Autodesk Fusion 360 part; units mm, degrees
sketch "Skizze1" plane through (0, 0, 0) normal (0, 1, 0) x (1, 0, 0)
  line L0 (13.5, -1) -> (-13.5, -1)
  line L1 (-13.5, -1) -> (-13.5, 0)
  line L2 (-13.5, 0) -> (13.5, 0)
  line L3 (13.5, 0) -> (13.5, -1)
  line L4 (13.5, -1) -> (-13.5, 0) construction
  line L5 (-13.5, -1) -> (13.5, 0) construction
  line L6 (-13.5, 0) -> (-12.5, 0)
  line L7 (-12.5, 0) -> (-12.5, -7.5)
  line L8 (-12.5, -7.5) -> (-13.5, -7.5)
  line L9 (-13.5, -7.5) -> (-13.5, 0)
  line L10 (13.5, 0) -> (12.5, 0)
  line L11 (12.5, 0) -> (12.5, -7.5)
  line L12 (12.5, -7.5) -> (13.5, -7.5)
  line L13 (13.5, -7.5) -> (13.5, 0)
  line L14 (-12.5, -7.5) -> (-17.5, -7.5)
  line L15 (-17.5, -7.5) -> (-17.5, -6.5)
  line L16 (-17.5, -6.5) -> (-12.5, -6.5)
  line L17 (-12.5, -6.5) -> (-12.5, -7.5)
  line L18 (12.5, -7.5) -> (17.5, -7.5)
  line L19 (17.5, -7.5) -> (17.5, -6.5)
  line L20 (17.5, -6.5) -> (12.5, -6.5)
  line L21 (12.5, -6.5) -> (12.5, -7.5)
  point P0 (0, -0.5)
  dimension "d7" = 27
  dimension "d8" = 1
  dimension "d9" = 7.5
  dimension "d10" = 1
  dimension "d11" = 7.5
  dimension "d12" = 1
  dimension "d13" = 5
  dimension "d14" = 1
  dimension "d15" = 5
  dimension "d16" = 1
extrude "Extrusion1" add sketch "Skizze1" along normal blind 100
fillet "Abrundung1" radius 1.5 4 edges at (12.5, 50, 7.5) (-12.5, 50, 7.5) (13.5, 50, 0) (-13.5, 50, 0)
fillet "Abrundung2" radius 0.5 4 edges at (-13.5, 50, 6.5) (13.5, 50, 6.5) (12.5, 50, 1) (-12.5, 50, 1)
sketch "Skizze2" plane through (0, 0, 1) normal (0, 0, 1) x (-1, 0, 0)
  line L0 (12, -100) -> (12, 0)
  line L1 (12, 0) -> (-12, 0)
  line L2 (-12, 0) -> (-12, -100)
  line L3 (-12, -100) -> (12, -100)
  line L4 (0, 0) -> (0, -3.5) construction
  line L5 (-2.6, -6.1) -> (-2.6, -18.9)
  arc A0 (-2.6, -18.9) -> (2.6, -18.9) centre (0, -18.9) ccw
  line L6 (2.6, -18.9) -> (2.6, -6.1)
  arc A1 (2.6, -6.1) -> (-2.6, -6.1) centre (0, -6.1) ccw
  line L7 (0, -3.5) -> (0, -21.5) construction
  point P0 (0, -3.5)
  dimension "d26" = 3.5
  dimension "d34" = 18
  dimension "d35" = 5.2
extrude "Extrusion2" cut sketch "Skizze2" against normal blind 1 contours L5 A0 L6 A1
pattern_linear "R-Anordnung1" count 4 spacing 25 along (0, 1, 0) of "Extrusion2"
equation "InnerWidth = 27 mm"
equation "OuterWidth = 37 mm"
equation "Height = 7.5 mm"
equation "Thickness = 1 mm"
equation "Length = 100 mm"
equation "SlotDistance = 25 mm"
equation "d7 = InnerWidth"
equation "d8 = Thickness"
equation "d9 = Height"
equation "d10 = Thickness"
equation "d11 = Height"
equation "d12 = Thickness"
equation "d13 = ( OuterWidth - InnerWidth ) / 2"
equation "d14 = Thickness"
equation "d15 = ( OuterWidth - InnerWidth ) / 2"
equation "d16 = Thickness"
equation "d17 = Length"
equation "OuterFillet = 1.5 mm"
equation "d20 = OuterFillet"
equation "InnerFillet = OuterFillet - Thickness"
equation "d22 = InnerFillet"
equation "SlotWidth = 5.2 mm"
equation "SlotLength = 18 mm"
equation "SlotDistance2 = 25 mm"
equation "d26 = Linear Dimension-2"
equation "d30 = Length / SlotDistance2"
equation "d32 = SlotDistance2"
equation "d34 = SlotLength"
equation "d35 = SlotWidth"
Model file for the job. Use its own axes, mm. A direction names the side the tool comes from. Round coordinates to 2 decimals unless told otherwise and drop trailing zeros. Order: outer loops, then holes, each group sorted by start corner. A loop starts at its lowest first (then second) coordinate and runs counter-clockwise, first axis right, second up.
(1) Band-saw the part on B-B (y = 42). List the corners of the cut face in (x, z).
(2) 3-axis set-ups, long thin cutter, end or side, ignore diameter. For faces 1 (the face through (16, 49, 6.5)), 2 (the face through (-13.5, 49, 4)), 3 (the face through (-0.1, 28.5, 0.5)): which of +Z, -Z, +X, -X, +Y, -Y reach the whole face in a straight line?
(3) Pull direction Y, two halves, no side cores. Call faces 4 (the face through (0.1, 96.5, 0.5)), 5 (the face through (-0.1, 0, 0.4)), 6 (the face through (12.5, 49, 4)): released by +Y, released by -Y, zero draft, split by the parting line, or undercut.
(4) Band-saw the part on C-C (x = 0). List the corners of the cut face in (y, z).
(5) Drill centre lines: line 1 (X direction, y = 55, z = 3.75); line 2 (Z direction, x = -6.5, y = 94); line 3 (X direction, y = 90, z = 1.25). Where is each one in solid material? Low to high.
(6) Pin check, flat tips, straight feed: pin 1 (0.5 mm diameter, centred on y = 13.5, z = 0.5, fed in from +X); pin 2 (3.5 mm diameter, centred on y = 51.5, z = 4, fed in from -X); pin 3 (2 mm diameter, centred on y = 49.5, z = 4, fed in from +X); pin 4 (12 mm diameter, centred on x = 13, y = 17.5, fed in from -Z). Stop position of each tip, or through.
(7) Band-saw the part on A-A (z = 5). List the corners of the cut face in (x, y), then the cut area to 3 significant figures.
(8) Band-saw the part on D-D (y = 73). List the corners of the cut face in (x, z).
Verdict:
1. outline: (-17.5, 6.5) - (-14, 6.5) arc R0.5 cw to (-13.5, 6) - (-13.5, 1.5) arc R1.5 ccw to (-12, 0) - (-2.6, 0) - (-2.6, 1) - (-12, 1) arc R0.5 cw to (-12.5, 1.5) - (-12.5, 6) arc R1.5 ccw to (-14, 7.5) - (-17.5, 7.5) - close; (2.6, 0) - (12, 0) arc R1.5 ccw to (13.5, 1.5) - (13.5, 6) arc R0.5 cw to (14, 6.5) - (17.5, 6.5) - (17.5, 7.5) - (14, 7.5) arc R1.5 ccw to (12.5, 6) - (12.5, 1.5) arc R0.5 cw to (12, 1) - (2.6, 1) - close
2. face 1: -Z, +X, +Y, -Y
2. face 2: -Z, -X, +Y, -Y
2. face 3: +Z, -Z
3. face 4: undercut
3. face 5: released by -Y
3. face 6: zero draft
4. outline: (0, 0) - (3.5, 0) - (3.5, 1) - (0, 1) - close; (21.5, 0) - (28.5, 0) - (28.5, 1) - (21.5, 1) - close; (46.5, 0) - (53.5, 0) - (53.5, 1) - (46.5, 1) - close; (71.5, 0) - (78.5, 0) - (78.5, 1) - (71.5, 1) - close; (96.5, 0) - (100, 0) - (100, 1) - (96.5, 1) - close
5. line 1: x = -13.5 to -12.5, 12.5 to 13.5
5. line 2: z = 0 to 1
5. line 3: x = -13.48 to -12.43, 12.43 to 13.48
6. pin 1: stops at x = 13.3
6. pin 2: stops at x = -13.5
6. pin 3: stops at x = 13.5
6. pin 4: stops at z = 0
7. outline: (-13.5, 0) - (-12.5, 0) - (-12.5, 100) - (-13.5, 100) - close; (12.5, 0) - (13.5, 0) - (13.5, 100) - (12.5, 100) - close
7. area: 200 mm2
8. outline: (-17.5, 6.5) - (-14, 6.5) arc R0.5 cw to (-13.5, 6) - (-13.5, 1.5) arc R1.5 ccw to (-12, 0) - (12, 0) arc R1.5 ccw to (13.5, 1.5) - (13.5, 6) arc R0.5 cw to (14, 6.5) - (17.5, 6.5) - (17.5, 7.5) - (14, 7.5) arc R1.5 ccw to (12.5, 6) - (12.5, 1.5) arc R0.5 cw to (12, 1) - (-12, 1) arc R0.5 cw to (-12.5, 1.5) - (-12.5, 6) arc R1.5 ccw to (-14, 7.5) - (-17.5, 7.5) - close
